Source: CAD feature listing. Evaluate the final solid. Frame: model axes, mm. A direction names the side the tool comes from. Round coordinates to 2 decimals unless told otherwise and drop trailing zeros. Order: outer loops, then holes, each group sorted by start corner. A loop starts at its lowest first (then second) coordinate and runs counter-clockwise, first axis right, second up. Notation, with made-up numbers: M -39,-5 L -33,-5 A13 ccw -33,19 Z; hole C -35.5,1.25 d2. An arc over 180 degrees is marked long. Answer in a Markdown table with one row per item. Add a question column.
```python
from build123d import *

# Parameters (mm, degrees)
F0_R     = 34.5
F1_DEPTH = 19
F2_R     = 22.5
F3_DEPTH = 6
F4_R     = 30
F5_DEPTH = 3
F6_R     = 19
F7_DEPTH = 28


with BuildPart() as f1:
    # F0 (on Front) → F1 (new body)
    with BuildSketch(Plane.XZ):
        Circle(F0_R)
    extrude(amount=-F1_DEPTH)

    # F2 (on face) → F3 (join)
    with BuildSketch(Plane.XZ):
        Circle(F2_R)
    extrude(amount=F3_DEPTH)

    # F4 (on face) → F5 (join)
    with BuildSketch(Plane(origin=(0, 19, 0), x_dir=(-1, 0, 0), z_dir=(0, 1, 0))):
        Circle(F4_R)
    extrude(amount=F5_DEPTH)

    # F6 (on face) → F7 (cut)
    with BuildSketch(Plane.XZ.offset(6)):
        Circle(F6_R)
    extrude(amount=-F7_DEPTH, mode=Mode.SUBTRACT)


solid = f1.part
```
(1) Draft query along X for faces 4 (the face through (8.767, 7.804, -16.856)), 5 (the face through (32.907, 9.367, 10.363)), 6 (the face through (0, 0, -23)). Return one class per face: +X half, -X half, draft (parallel to the pull), parting line (faces both ways), or undercut.
(2) Access query for faces 1 (the face through (29.97, 20.48, 1.32)), 2 (the face through (10.382, -2.958, -19.961)), 3 (the face through (-15, -6, -12)). Directions: +Z, -Z, +X, -X, +Y, -Y. A direction counts if a zero-diameter tool reaches every point of the face in a straight line with its end or side. Return the directions, or none.
(3) Cut plane B-B (x = 0). Return loops of the section in (y, z).
(4) Line query: line 1 (Z direction, x = 0, y = 14.75); line 2 (Z direction, x = 0.5, y = -2.75); line 3 (Y direction, x = 8.5, z = 25). Output: solid intervals per line, ascending. Write a range as from..to.
(5) Cut plane D-D (x = -27). Return loops of the section in (y, z), and give its area (3 significant figures).
(6) Cut plane A-A (z = 0). Return loops of the section in (x, y).
(7) Cut plane C-C (y = 5). Return loops of the section in (x, z).
(8) Pin query (flat end, axial travel): pin 1 (4 mm diameter, centred on x = -12.5, y = 19, fed in from -Z); pin 2 (6 mm diameter, centred on y = 18, z = -4.5, fed in from +X); pin 3 (12 mm diameter, centred on x = -26.5, y = -0.5, fed in from +Z). Return the tip coordinate at first contact, or that it passes through.
Answer list:
| question | item | result |
|---|---|---|
| 1 | face 4 | undercut |
| 1 | face 5 | parting line |
| 1 | face 6 | draft |
| 2 | face 1 | +Y |
| 2 | face 2 | -Y |
| 2 | face 3 | +Z, -Z, +X, -X, -Y |
| 3 | outline | M -6,-22.5 L 0,-22.5 L 0,-34.5 L 19,-34.5 L 19,-30 L 22,-30 L 22,-19 L -6,-19 Z; M -6,19 L 22,19 L 22,30 L 19,30 L 19,34.5 L 0,34.5 L 0,22.5 L -6,22.5 Z |
| 4 | line 1 | -34.5..-19, 19..34.5 |
| 4 | line 2 | -22.49..-18.99, 18.99..22.49 |
| 4 | line 3 | 0..22 |
| 5 | outline | M 0,-21.48 L 19,-21.48 L 19,-13.08 L 22,-13.08 L 22,13.08 L 19,13.08 L 19,21.48 L 0,21.48 Z |
| 5 | area | 895 mm² |
| 6 | outline | M -34.5,0 L -22.5,0 L -22.5,-6 L -19,-6 L -19,22 L -30,22 L -30,19 L -34.5,19 Z; M 19,-6 L 22.5,-6 L 22.5,0 L 34.5,0 L 34.5,19 L 30,19 L 30,22 L 19,22 Z |
| 7 | outline | C 0,0 d69; hole C 0,0 d38 |
| 8 | pin 1 | z = -32.86 |
| 8 | pin 2 | x = 34.47 |
| 8 | pin 3 | z = 27.73 |
